Can you work these out from the model? Positions are in its coordinate system, mm. A direction names the side the tool comes from. Give positions to 0.01 mm unless a question says otherwise; leave off trailing zeros. Loops run counter-clockwise (first coordinate to the right, second up) from the corner with the lowest first, then second, coordinate; pieces in that order, holes last. Notation, with made-up numbers: (13.25, -24.5) -> (29.25, -24.5) arc R12 ccw to (29.25, -16.5) -> close; hole circle Ø2 at (-8.5, -5). An arc over 180 degrees is marked (long way). One line per question, with ' | ' between items.
from build123d import *

# Parameters (mm, degrees)
SKETCH_1_W      = 10
SKETCH_1_H      = 9.6
SKETCH_1_R      = 2
SKETCH_1_W_2    = 9.6
SKETCH_1_H_2    = 10
SKETCH_1_R_2    = 4
EXTRUDE_2_DEPTH = 3
SKETCH_2_R      = 3.95
EXTRUDE_3_DEPTH = 120


with BuildPart() as part:
    # 草图1 → 凸台-拉伸2 (new body)
    # profile 1 of 6: a face of its own
    with BuildSketch(Plane(origin=(0, 0, 0), x_dir=(1, 0, 0), z_dir=(0, 1, 0))):
        with Locations((-9.8, 0)):
            Rectangle(SKETCH_1_W, SKETCH_1_H)
        with Locations(Location((-9.946440474, 0.053559526, 0), (0, 0, 270))):
            Circle(SKETCH_1_R, mode=Mode.SUBTRACT)
    # profile 2 of 6: a face of its own
    with BuildSketch(Plane(origin=(0, 0, 0), x_dir=(1, 0, 0), z_dir=(0, 1, 0))):
        with Locations((0, -9.8)):
            Rectangle(SKETCH_1_W_2, SKETCH_1_H_2)
        with Locations(Location((-0.053559526, -9.946440474, 0), (0, 0, 270))):
            Circle(SKETCH_1_R, mode=Mode.SUBTRACT)
    # profile 3 of 6: a face of its own
    with BuildSketch(Plane(origin=(0, 0, 0), x_dir=(1, 0, 0), z_dir=(0, 1, 0))):
        Rectangle(SKETCH_1_W_2, SKETCH_1_H)
        Circle(SKETCH_1_R_2, mode=Mode.SUBTRACT)
    # profile 4 of 6: a face of its own
    with BuildSketch(Plane(origin=(0, 0, 0), x_dir=(1, 0, 0), z_dir=(0, 1, 0))):
        with Locations((9.8, 0)):
            Rectangle(SKETCH_1_W, SKETCH_1_H)
        with Locations(Location((9.946440474, -0.053559526, 0), (0, 0, 270))):
            Circle(SKETCH_1_R, mode=Mode.SUBTRACT)
    # profile 5 of 6: a face of its own
    with BuildSketch(Plane(origin=(0, 0, 0), x_dir=(1, 0, 0), z_dir=(0, 1, 0))):
        with Locations((0, 9.8)):
            Rectangle(SKETCH_1_W_2, SKETCH_1_H_2)
        with Locations(Location((0.053559526, 9.946440474, 0), (0, 0, 270))):
            Circle(SKETCH_1_R, mode=Mode.SUBTRACT)
    # profile 6 of 6: a face of its own
    with BuildSketch(Plane(origin=(0, 0, 0), x_dir=(1, 0, 0), z_dir=(0, 1, 0))):
        Circle(SKETCH_1_R_2)
    extrude(amount=EXTRUDE_2_DEPTH)

    # 草图2 → 凸台-拉伸3 (add)
    with BuildSketch(Plane(origin=(0, 3, 0), x_dir=(1, 0, 0), z_dir=(0, 1, 0))):
        with Locations(Location((0, 0, 0), (0, 0, 270))):
            Circle(SKETCH_2_R)
    extrude(amount=EXTRUDE_3_DEPTH)


solid = part.part
Q1. If we mould it in two halves opening along X, with no side actions, what happens to faces 1 (the face through (-0.71, 1.48, -8.1)), 2 (the face through (10, 1, 4.8)), 3 (the face through (-1.27, 1.48, 8.36)), 4 (the face through (-14.8, 1, 0))? For each: pulls with the +X half, pulls with the -X half, needs draft (parallel to the pull), parting line crosses it, or undercut.
Entries:
face 1: undercut | face 2: needs draft | face 3: undercut | face 4: pulls with the -X half
Q2. On a 3-axis mill with a long thin cutter (end or side, diameter ignored), from which of +Z, -Z, +X, -X, +Y, -Y can I reach the whole of each face in a straight line? I mean faces 5 (the face through (10, 1, -4.8)), 6 (the face through (-4.8, 1, 10)), 7 (the face through (-10, 1, -4.8)), 8 (the face through (-3, 3, -3)). Say none if no direction works.
Entries:
face 5: -Z, +X, +Y, -Y | face 6: +Z, -X, +Y, -Y | face 7: -Z, -X, +Y, -Y | face 8: +Y
Q3. If I drill on probe 1 along Y at (x, z) = (-2.5, 4.75); probe 2 along Z at (x, y) = (0.75, 73.5); probe 3 along X at (y, z) = (95, 1.5), over which ranges is the centre line in solid material (lowest first)? Write a range as from..to.
Entries:
probe 1: 0..3 | probe 2: -3.88..3.88 | probe 3: -3.65..3.65
Q4. For pin 1 Ø1.5 at (y, z) = (1.5, -11) entering from +X; pin 2 Ø3.5 at (x, y) = (11.5, 2) entering from +Z; pin 3 Ø1 at (y, z) = (63, 3) entering from +X, each with a flat end and sliding along its axis, tell me the tip position at first contact or that it passes through.
Entries:
pin 1: x = 4.8 | pin 2: z = 4.8 | pin 3: x = 3.06
Q5. If we section it at B-B (z = -9.5): Write out the boundary of the cut face in (x, y), plus the area to 3 significant figures.
Entries:
outline: (-4.8, 0) -> (-1.9, 0) -> (-1.9, 3) -> (-4.8, 3) -> close; (2, 0) -> (4.8, 0) -> (4.8, 3) -> (2, 3) -> close | area: 17.1 mm²
Q6. If we section it at C-C (y = 41): Write out the boundary of the cut face in (x, z).
Entries:
outline: circle Ø7.9 at (0, 0)
Q7. If we section it at A-A (z = 0): Write out the boundary of the cut face in (x, y).
Entries:
outline: (-14.8, 0) -> (-11.95, 0) -> (-11.95, 3) -> (-14.8, 3) -> close; (-7.95, 0) -> (7.95, 0) -> (7.95, 3) -> (3.95, 3) -> (3.95, 123) -> (-3.95, 123) -> (-3.95, 3) -> (-7.95, 3) -> close; (11.95, 0) -> (14.8, 0) -> (14.8, 3) -> (11.95, 3) -> close
